For this review, use the dimensioned drawing (mm, ordinates from the lowest corner) and the shaded views. A direction names the side the tool comes from. Coordinates: 2 decimals unless noted, no trailing zeros. Write each loop counter-clockwise with the first axis right and the second up, starting at its lowest first coordinate (ties: lowest second). Pieces come first, ordered by that corner, then holes. Notation, with made-up numbers: M 57.25,-26.5 L 76.25,-26.5 A10 cw 76.25,-8.5 Z; hole C 89.25,6 d3. An arc over 180 degrees is marked long. One line per question, with ' | ' between items.
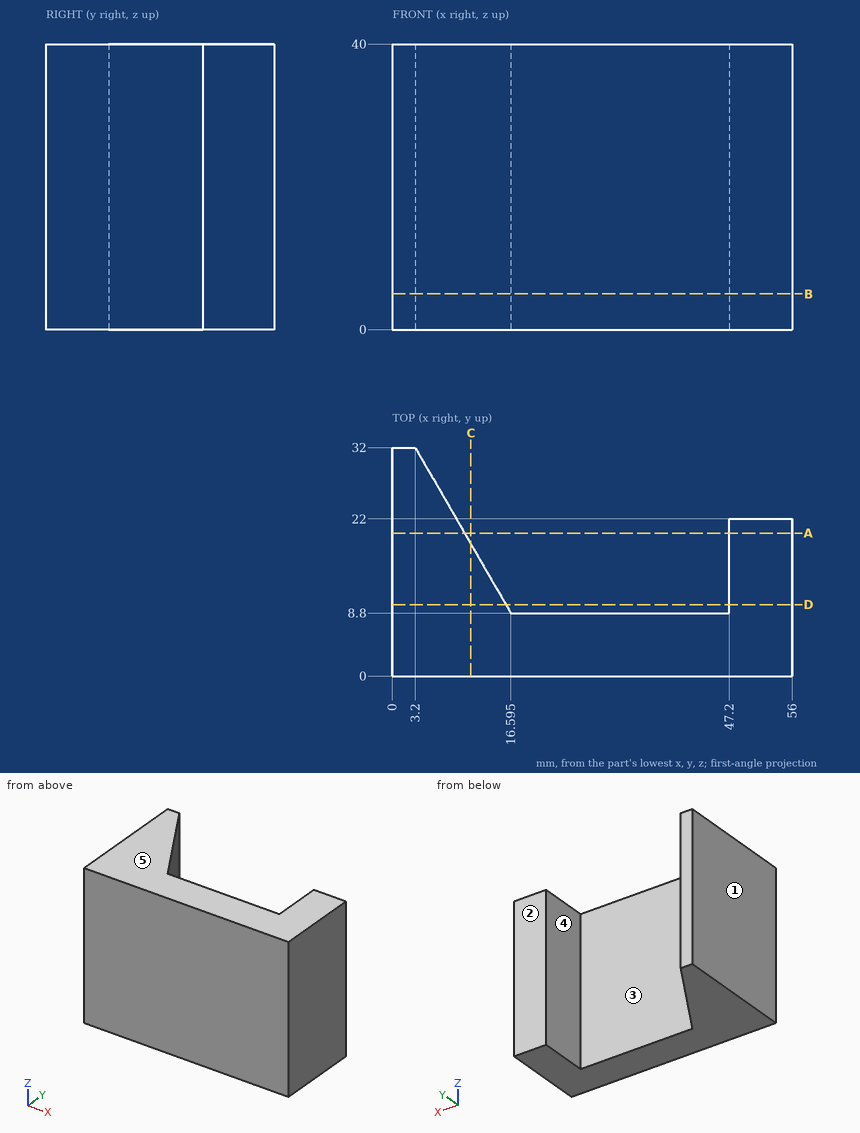
1. Take a section at B-B (z = 5). Write out the cut boundary in (x, y) (1 decimal).
Answer sheet:
outline: M 0,0 L 56,0 L 56,22 L 47.2,22 L 47.2,8.8 L 16.6,8.8 L 3.2,32 L 0,32 Z
2. Take a section at A-A (y = 20). Write out the cut boundary in (x, z).
Answer sheet:
outline: M 0,0 L 10.13,0 L 10.13,40 L 0,40 Z; M 47.2,0 L 56,0 L 56,40 L 47.2,40 Z
3. Take a section at D-D (y = 10). Write out the cut boundary in (x, z).
Answer sheet:
outline: M 0,0 L 15.9,0 L 15.9,40 L 0,40 Z; M 47.2,0 L 56,0 L 56,40 L 47.2,40 Z
4. Take a section at C-C (x = 11). Write out the cut boundary in (y, z).
Answer sheet:
outline: M 0,0 L 18.49,0 L 18.49,40 L 0,40 Z
5. To check wall thickness, follow line 1 along Y through (x, z) = (20, 8); line 2 along X through (y, z) = (19, 8.5) (1 decimal); line 3 along X through (y, z) = (17.5, 4). State the ranges of each line that lie inside material, in increasing order. Write a range as [from, to].
Answer sheet:
line 1: [0, 8.8] | line 2: [0, 10.7], [47.2, 56] | line 3: [0, 11.57], [47.2, 56]
6. Tool access review of the marked faces 4 and 5: name each direction out of +Z, -Z, +X, -X, +Y, -Y from which nothing blocks a thin tool from reaching the whole face with its end or side.
Answer sheet:
face 4: +Z, -Z, +Y | face 5: +Z, +X, -X, +Y, -Y
7. Draft analysis for pull direction X (two halves, no side actions). For the marked faces 1, 2 and 3, state which applies: pulls with the +X half, pulls with the -X half, needs draft (parallel to the pull), parting line crosses it, or undercut.
Answer sheet:
face 1: pulls with the -X half | face 2: needs draft | face 3: undercut
8. Insertion check: pin 1 Ø6 at (y, z) = (28, 7) entering from +X; pin 2 Ø1 at (x, z) = (33.5, 7.5) entering from +Y; pin 3 Ø7 at (x, z) = (50.5, 17) entering from +Y. Each pin has a flat end and moves straight along its axis. Give the tip position at first contact, or say it passes through.
Answer sheet:
pin 1: x = 7.24 | pin 2: y = 8.8 | pin 3: y = 22
